from build123d import *

# Parameters (mm, degrees)
BOSS_EXTRUDE1_DEPTH = 1.5
BOSS_EXTRUDE2_DEPTH = 1.5
SKETCH4_R           = 2.5
BOSS_EXTRUDE3_DEPTH = 3
FILLET1_R           = 0.5


with BuildPart() as part:
    # Sketch2 → Boss-Extrude1 (new body)
    with BuildSketch(Plane(origin=(0, 0, 0), x_dir=(1, 0, 0), z_dir=(0, 1, 0))):
        with BuildLine():
            Line((-25.815069681, 36.858949759), (0, 0))
            Line((0, 0), (27.07764911, 35.94163211))
            ThreePointArc((27.07764911, 35.94163211), (0.780317, 44.993233996), (-25.815069681, 36.858949759))
        make_face()
    extrude(amount=BOSS_EXTRUDE1_DEPTH)

    # Sketch3 → Boss-Extrude2 (add)
    with BuildSketch(Plane.XZ):
        with BuildLine():
            Line((0, -34.375), (10, -34.375))
            ThreePointArc((10, -34.375), (10.625, -35), (10, -35.625))
            Line((10, -35.625), (0, -35.625))
            ThreePointArc((0, -35.625), (-0.625, -35), (0, -34.375))
        make_face()
    extrude(amount=BOSS_EXTRUDE2_DEPTH)

    # Sketch4 → Boss-Extrude3 (add)
    with BuildSketch(Plane(origin=(0, 1.5, 0), x_dir=(1, 0, 0), z_dir=(0, 1, 0))):
        with Locations((0, 35)):
            Circle(SKETCH4_R)
    extrude(amount=BOSS_EXTRUDE3_DEPTH)

    # Fillet1
    fillet1_edges = [part.edges().sort_by_distance(p)[0] for p in [
        (-2.5, 4.5, -35),
    ]]
    fillet(fillet1_edges, radius=FILLET1_R)


solid = part.part
Geometry: final body of the model. Coordinates: model frame, mm. A direction names the side the tool comes from. Coordinates: 2 decimals unless noted, no trailing zeros. Order: outer loops, then holes, each group sorted by start corner. A loop starts at its lowest first (then second) coordinate and runs counter-clockwise, first axis right, second up.
1) Section B-B (x = 3.5). Return loops of the section in (y, z) (3 decimals), then the cut area to 3 significant figures.
Result sheet:
outline: (-1.5, -35.625) - (0, -35.625) - (0, -44.864) - (1.5, -44.864) - (1.5, -4.646) - (0, -4.646) - (0, -34.375) - (-1.5, -34.375) - close
area: 62.2 mm2
2) Section D-D (y = 0.7). Return loops of the section in (x, z), then the cut area to 3 significant figures.
Result sheet:
outline: (-25.82, -36.86) arc R45 ccw to (27.08, -35.94) - (0, 0) - close
area: 1,270 mm2
3) Section A-A (y = 3.4). Return loops of the section in (x, z), then the cut area to 3 significant figures.
Result sheet:
outline: circle Ø5 at (0, -35)
area: 19.6 mm2
4) Section C-C (z = -35). Return loops of the section in (x, y) (3 decimals), then the cut area to 3 significant figures.
Result sheet:
outline: (-24.513, 0) - (-0.625, 0) - (-0.625, -1.5) - (10.625, -1.5) - (10.625, 0) - (26.368, 0) - (26.368, 1.5) - (2.5, 1.5) - (2.5, 4) arc R0.5 ccw to (2, 4.5) - (-2, 4.5) arc R0.5 ccw to (-2.5, 4) - (-2.5, 1.5) - (-24.513, 1.5) - close
area: 108 mm2
5) First-contact query: P1, Ø1.5, axis at x = 9, y = 0.5, coming from the -Z side; P2, Ø12, axis at x = -19, z = -21, coming from the +Y side; P3, Ø22.5, axis at x = -12.5, z = -30, coming from the +Y side. Flat tips, straight axial feed; report the tip coordinate or a pass-through.
Result sheet:
P1: stops at z = -44.24
P2: stops at y = 1.5
P3: stops at y = 4.45
6) Ray query, probe 1 along Z at (x, y) = (4.5, -0.55) (3 decimals); probe 2 along Y at (x, z) = (7, -21); probe 3 along X at (y, z) = (2.45, -35). Return the intervals inside material, ascending.
Result sheet:
probe 1: z = -35.625 to -34.375
probe 2: y = 0 to 1.5
probe 3: x = -2.5 to 2.5
7) Set-up query: faces 1 (the cylindrical face through (-0.625, -0.74, -35.014)), 2 (the cylindrical face through (-0.54, 2.73, -32.56)), 3 (the flat face through (5, -1, -35.625)), 4 (the flat face through (5, -1, -34.375)). Return all of +Z, -Z, +X, -X, +Y, -Y with unobstructed straight access to the full face (end or side cutting, diameter ignored); none if empty.
Result sheet:
face 1: -X, -Y
face 2: +Y
face 3: -Z, +X, -X, -Y
face 4: +Z, +X, -X, -Y
